from build123d import *

# Parameters (mm, degrees)
F0_R     = 3.429
F1_DEPTH = 9.525
F2_SIZE  = 2.54


with BuildPart() as f1:
    # F0 (on Top) → F1 (new body)
    with BuildSketch(Plane.XY):
        with BuildLine():
            Line((-117.757219, 148.59), (-240.312219, 148.59))
            ThreePointArc((-240.312219, 148.59), (-252.82932, 138.037595), (-244.545552, 123.916325))
            ThreePointArc((-244.545552, 123.916325), (-241.477465, 121.595662), (-240.312219, 117.929488))
            Line((-240.312219, 117.929488), (-240.312219, 30.660512))
            ThreePointArc((-240.312219, 30.660512), (-241.477465, 26.994338), (-244.545552, 24.673675))
            ThreePointArc((-244.545552, 24.673675), (-252.82932, 10.552405), (-240.312219, 0))
            Line((-240.312219, 0), (-117.757219, 0))
            Line((-117.757219, 0), (-117.757219, 12.7))
            Line((-117.757219, 12.7), (-145.062219, 12.7))
            ThreePointArc((-145.062219, 12.7), (-149.552347, 14.559872), (-151.412219, 19.05))
            Line((-151.412219, 19.05), (-151.412219, 129.54))
            ThreePointArc((-151.412219, 129.54), (-149.552347, 134.030128), (-145.062219, 135.89))
            Line((-145.062219, 135.89), (-117.757219, 135.89))
            Line((-117.757219, 135.89), (-117.757219, 148.59))
        make_face()
        with Locations((-240.312219, 12.7)):
            Circle(F0_R, mode=Mode.SUBTRACT)
        with BuildLine():
            ThreePointArc((-227.612219, 129.54), (-225.752347, 134.030128), (-221.262219, 135.89))
            Line((-221.262219, 135.89), (-166.652219, 135.89))
            ThreePointArc((-166.652219, 135.89), (-162.162091, 134.030128), (-160.302219, 129.54))
            Line((-160.302219, 129.54), (-160.302219, 19.05))
            ThreePointArc((-160.302219, 19.05), (-162.162091, 14.559872), (-166.652219, 12.7))
            Line((-166.652219, 12.7), (-221.262219, 12.7))
            ThreePointArc((-221.262219, 12.7), (-225.752347, 14.559872), (-227.612219, 19.05))
            Line((-227.612219, 19.05), (-227.612219, 129.54))
        make_face(mode=Mode.SUBTRACT)
        with Locations((-240.312219, 135.89)):
            Circle(F0_R, mode=Mode.SUBTRACT)
        with BuildLine():
            Line((4.797781, 148.59), (-117.757219, 148.59))
            Line((-117.757219, 148.59), (-117.757219, 135.89))
            Line((-117.757219, 135.89), (-90.452219, 135.89))
            ThreePointArc((-90.452219, 135.89), (-85.962091, 134.030128), (-84.102219, 129.54))
            Line((-84.102219, 129.54), (-84.102219, 19.05))
            ThreePointArc((-84.102219, 19.05), (-85.962091, 14.559872), (-90.452219, 12.7))
            Line((-90.452219, 12.7), (-117.757219, 12.7))
            Line((-117.757219, 12.7), (-117.757219, 0))
            Line((-117.757219, 0), (4.797781, 0))
            ThreePointArc((4.797781, 0), (17.314883, 10.552405), (9.031115, 24.673675))
            ThreePointArc((9.031115, 24.673675), (5.963028, 26.994338), (4.797781, 30.660512))
            Line((4.797781, 30.660512), (4.797781, 117.929488))
            ThreePointArc((4.797781, 117.929488), (5.963028, 121.595662), (9.031115, 123.916325))
            ThreePointArc((9.031115, 123.916325), (17.314883, 138.037595), (4.797781, 148.59))
        make_face()
        with Locations((4.797781, 12.7)):
            Circle(F0_R, mode=Mode.SUBTRACT)
        with BuildLine():
            Line((-7.902219, 129.54), (-7.902219, 19.05))
            ThreePointArc((-7.902219, 19.05), (-9.762091, 14.559872), (-14.252219, 12.7))
            Line((-14.252219, 12.7), (-68.862219, 12.7))
            ThreePointArc((-68.862219, 12.7), (-73.352347, 14.559872), (-75.212219, 19.05))
            Line((-75.212219, 19.05), (-75.212219, 129.54))
            ThreePointArc((-75.212219, 129.54), (-73.352347, 134.030128), (-68.862219, 135.89))
            Line((-68.862219, 135.89), (-14.252219, 135.89))
            ThreePointArc((-14.252219, 135.89), (-9.762091, 134.030128), (-7.902219, 129.54))
        make_face(mode=Mode.SUBTRACT)
        with Locations((4.797781, 135.89)):
            Circle(F0_R, mode=Mode.SUBTRACT)
    extrude(amount=F1_DEPTH)

    # F2
    f2_edges = [f1.edges().sort_by_distance(p)[0] for p in [
        (-117.757219, 0, 9.525),
    ]]
    chamfer(f2_edges, length=F2_SIZE)


solid = f1.part
Build history of the part. All positions in model axes, mm. A direction names the side the tool comes from. Coordinates: 2 decimals unless noted, no trailing zeros. Write each loop counter-clockwise with the first axis right and the second up, starting at its lowest first coordinate (ties: lowest second). Pieces come first, ordered by that corner, then holes.
(1) Mould opens along Y. For faces 4 (the flat face through (-119, 0, 3)), 5 (the flat face through (-194, 12.7, 5)), 6 (the flat face through (-120, 139, 9.525)) say: pulls with the +Y half, pulls with the -Y half, needs draft (parallel to the pull), parting line crosses it, or undercut.
(2) Drill centre lines: line 1 (X direction, y = 79.5, z = 4.5); line 2 (X direction, y = 137, z = 1.5); line 3 (Y direction, x = -99.5, z = 5.25). Where is each one in solid material? Low to high.
(3) Cut at B-B on x = -54. List the corners of the cut face in (y, z) (3 decimals), and give its area (3 significant figures).
(4) Cut at C-C on z = 3.5. State how many separate pieces and enclosed holes the cut face has, and give its area (3 significant figures).
(5) 3-axis set-ups, long thin cutter, end or side, ignore diameter. For faces 1 (the flat face through (-41, 12.7, 5)), 2 (the cylindrical face through (-252.785, 138.283, 3.444)), 3 (the cylindrical face through (5.995, 26.95, 3.444)): which of +Z, -Z, +X, -X, +Y, -Y reach the whole face in a straight line?
(6) Cut at A-A on y = 78.5. List the corners of the cut face in (x, z) (3 decimals).
(7) Pin check, flat tips, straight feed: pin 1 Ø6 at (x, y) = (4.8, 135.89) entering from -Z; pin 2 Ø3 at (y, z) = (58, 5.5) entering from -X; pin 3 Ø5 at (y, z) = (18.5, 8.5) entering from -X; pin 4 Ø3 at (y, z) = (126, 4.5) entering from -X. Stop position of each tip, or through.
Working result:
1. face 4: pulls with the -Y half
1. face 5: undercut
1. face 6: needs draft
2. line 1: x = -240.31 to -227.61, -160.3 to -151.41, -84.1 to -75.21, -7.9 to 4.8
2. line 2: x = -252.96 to -243.56, -237.07 to 1.55, 8.04 to 17.45
2. line 3: y = 0 to 12.7, 135.89 to 148.59
3. outline: (0, 0) - (12.7, 0) - (12.7, 9.525) - (2.54, 9.525) - (0, 6.985) - close; (135.89, 0) - (148.59, 0) - (148.59, 6.985) - (146.05, 9.525) - (135.89, 9.525) - close
3. area: 235 mm2
4. separate pieces: 1
4. enclosed holes: 7
4. area: 12,500 mm2
5. face 1: +Z, -Z
5. face 2: +Z, -Z, -X
5. face 3: +Z, -Z, +X
6. outline: (-240.312, 0) - (-227.612, 0) - (-227.612, 9.525) - (-237.772, 9.525) - (-240.312, 6.985) - close; (-160.302, 0) - (-151.412, 0) - (-151.412, 9.525) - (-160.302, 9.525) - close; (-84.102, 0) - (-75.212, 0) - (-75.212, 9.525) - (-84.102, 9.525) - close; (-7.902, 0) - (4.798, 0) - (4.798, 6.985) - (2.258, 9.525) - (-7.902, 9.525) - close
7. pin 1: passes through
7. pin 2: stops at x = -240.31
7. pin 3: stops at x = -252.43
7. pin 4: stops at x = -249.85
